Can you work these out from the model? Positions are in its coordinate system, mm. Face numbers are marked on the shaded views. A direction names the side the tool comes from. Coordinates: 2 decimals unless noted, no trailing zeros. Order: outer loops, then holes, each group sorted by start corner. A loop starts at its lowest first (then second) coordinate and runs counter-clockwise, first axis right, second up. Notation, with made-up numbers: (51, 4) -> (86, 4) arc R13 ccw to (86, 16) -> close; hole circle Ø8 at (33, 77.5). An arc over 180 degrees is marked (long way). Answer in a Markdown table with one row per item.
```python
from build123d import *

# Parameters (mm, degrees)
SKETCH1_W           = 80.5
SKETCH1_H           = 36.5
BOSS_EXTRUDE1_DEPTH = 1.6
SKETCH2_R           = 1.5
CUT_EXTRUDE1_DEPTH  = 1.6
SKETCH3_W           = 71.3
SKETCH3_H           = 26.799999994
BOSS_EXTRUDE2_DEPTH = 7.1
SKETCH4_R           = 0.5
CUT_EXTRUDE2_DEPTH  = 7.1
SKETCH5_W           = 64.5
SKETCH5_H           = 13.8
CUT_EXTRUDE3_DEPTH  = 1.5


with BuildPart() as part:
    # Sketch1 → Boss-Extrude1 (new body)
    with BuildSketch(Plane(origin=(0, 0, 0), x_dir=(1, 0, 0), z_dir=(0, 1, 0))):
        Rectangle(SKETCH1_W, SKETCH1_H)
    extrude(amount=BOSS_EXTRUDE1_DEPTH)

    # Sketch2 → Cut-Extrude1 (cut)
    with BuildSketch(Plane(origin=(0, 1.6, 0), x_dir=(1, 0, 0), z_dir=(0, 1, 0))):
        with Locations(Location((-37.75, 15.75, 0), (0, 0, 270))):
            Circle(SKETCH2_R)
        with Locations(Location((-37.75, -15.75, 0), (0, 0, 270))):
            Circle(SKETCH2_R)
        with Locations(Location((37.75, 15.75, 0), (0, 0, 270))):
            Circle(SKETCH2_R)
        with Locations(Location((37.75, -15.75, 0), (0, 0, 270))):
            Circle(SKETCH2_R)
    extrude(amount=-CUT_EXTRUDE1_DEPTH, mode=Mode.SUBTRACT)

    # Sketch3 → Boss-Extrude2 (add)
    with BuildSketch(Plane(origin=(0, 1.6, 0), x_dir=(1, 0, 0), z_dir=(0, 1, 0))):
        Rectangle(SKETCH3_W, SKETCH3_H)
    extrude(amount=BOSS_EXTRUDE2_DEPTH)

    # Sketch4 → Cut-Extrude2 (cut)
    with BuildSketch(Plane(origin=(0, 1.6, 0), x_dir=(1, 0, 0), z_dir=(0, 1, 0))):
        with Locations(Location((-32.25, 15.75, 0), (0, 0, 270))):
            Circle(SKETCH4_R)
        with Locations(Location((-29.71, 15.75, 0), (0, 0, 270))):
            Circle(SKETCH4_R)
        with Locations(Location((-27.17, 15.75, 0), (0, 0, 270))):
            Circle(SKETCH4_R)
        with Locations(Location((-24.63, 15.75, 0), (0, 0, 270))):
            Circle(SKETCH4_R)
        with Locations(Location((-22.09, 15.75, 0), (0, 0, 270))):
            Circle(SKETCH4_R)
        with Locations(Location((-19.55, 15.75, 0), (0, 0, 270))):
            Circle(SKETCH4_R)
        with Locations(Location((-17.01, 15.75, 0), (0, 0, 270))):
            Circle(SKETCH4_R)
        with Locations(Location((-14.47, 15.75, 0), (0, 0, 270))):
            Circle(SKETCH4_R)
        with Locations(Location((-11.93, 15.75, 0), (0, 0, 270))):
            Circle(SKETCH4_R)
        with Locations(Location((-9.39, 15.75, 0), (0, 0, 270))):
            Circle(SKETCH4_R)
        with Locations(Location((-6.85, 15.75, 0), (0, 0, 270))):
            Circle(SKETCH4_R)
        with Locations(Location((-4.31, 15.75, 0), (0, 0, 270))):
            Circle(SKETCH4_R)
        with Locations(Location((-1.77, 15.75, 0), (0, 0, 270))):
            Circle(SKETCH4_R)
        with Locations(Location((0.77, 15.75, 0), (0, 0, 270))):
            Circle(SKETCH4_R)
        with Locations(Location((3.31, 15.75, 0), (0, 0, 270))):
            Circle(SKETCH4_R)
        with Locations(Location((5.85, 15.75, 0), (0, 0, 270))):
            Circle(SKETCH4_R)
    extrude(amount=-CUT_EXTRUDE2_DEPTH, mode=Mode.SUBTRACT)

    # Sketch5 → Cut-Extrude3 (cut)
    with BuildSketch(Plane(origin=(0, 8.7, 0), x_dir=(1, 0, 0), z_dir=(0, 1, 0))):
        Rectangle(SKETCH5_W, SKETCH5_H)
    extrude(amount=-CUT_EXTRUDE3_DEPTH, mode=Mode.SUBTRACT)


solid = part.part
```
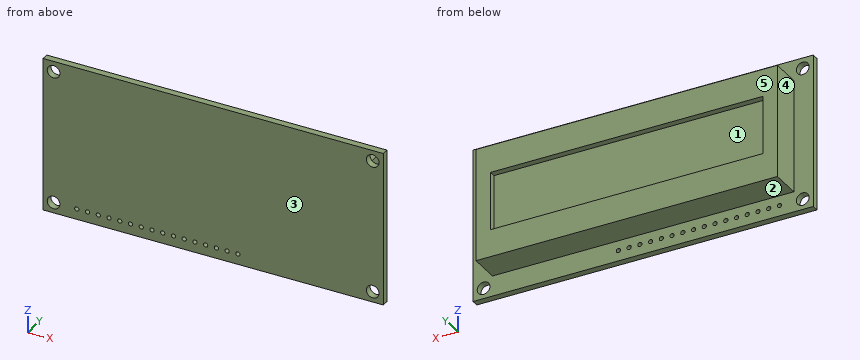
(1) Suppose I cut it at B-B (z = -10). Please give me the cut outline in (x, y), and give its area (3 significant figures).
Response values:
| item | result |
|---|---|
| outline | (-40.25, 0) -> (40.25, 0) -> (40.25, 1.6) -> (35.65, 1.6) -> (35.65, 8.7) -> (-35.65, 8.7) -> (-35.65, 1.6) -> (-40.25, 1.6) -> close |
| area | 635 mm2 |
(2) Suppose I cut it at A-A (x = -37.75). Please give me the cut outline in (y, z), and give its area (3 significant figures).
Response values:
| item | result |
|---|---|
| outline | (0, -18.25) -> (1.6, -18.25) -> (1.6, -17.25) -> (0, -17.25) -> close; (0, -14.25) -> (1.6, -14.25) -> (1.6, 14.25) -> (0, 14.25) -> close; (0, 17.25) -> (1.6, 17.25) -> (1.6, 18.25) -> (0, 18.25) -> close |
| area | 48.8 mm2 |
(3) Will these pins go through, and if not, where does the flat tip stop? pin 1 Ø5 at (y, z) = (6, 2) entering from -X; pin 2 Ø3.5 at (y, z) = (4, 4) entering from +X; pin 3 Ø2.5 at (x, z) = (-37.75, 15.75) entering from -Y; pin 4 Ø5 at (x, y) = (8, 7) entering from +Z.
Response values:
| item | result |
|---|---|
| pin 1 | x = -35.65 |
| pin 2 | x = 35.65 |
| pin 3 | through |
| pin 4 | z = 13.4 |
(4) Suppose I cut it at D-D (z = -6). Please give me the cut outline in (x, y), and give its area (3 significant figures).
Response values:
| item | result |
|---|---|
| outline | (-40.25, 0) -> (40.25, 0) -> (40.25, 1.6) -> (35.65, 1.6) -> (35.65, 8.7) -> (32.25, 8.7) -> (32.25, 7.2) -> (-32.25, 7.2) -> (-32.25, 8.7) -> (-35.65, 8.7) -> (-35.65, 1.6) -> (-40.25, 1.6) -> close |
| area | 538 mm2 |
(5) I need wall thicknesses on line 1 (X direction, y = 0.6, z = 15.75); line 2 (X direction, y = 7.75, z = -5); line 3 (Z direction, x = -0.5, y = 7.25). Which ranges of each line are inside material? Lowest first, please. Write a range as [from, to].
Response values:
| item | result |
|---|---|
| line 1 | [-40.25, -39.25], [-36.25, 36.25], [39.25, 40.25] |
| line 2 | [-35.65, -32.25], [32.25, 35.65] |
| line 3 | [-13.4, -6.9], [6.9, 13.4] |
(6) Suppose I cut it at C-C (y = 3). Please give me the cut outline in (x, z).
Response values:
| item | result |
|---|---|
| outline | (-35.65, -13.4) -> (35.65, -13.4) -> (35.65, 13.4) -> (-35.65, 13.4) -> close |
(7) On a 3-axis mill with a long thin cutter (end or side, diameter ignored), from which of +Z, -Z, +X, -X, +Y, -Y can I reach the whole of each face in a straight line? I mean the marked faces 4 and 5. Say none if no direction works.
Response values:
| item | result |
|---|---|
| face 4 | +Z, -Z, -X, +Y |
| face 5 | +Z, -Z, +X, -X, +Y |
(8) We'd pull the mould along Z, two halves only. Please class the marked faces 1, 2 and 3: +Z half, -Z half, draft (parallel to the pull), parting line (faces both ways), or undercut.
Response values:
| item | result |
|---|---|
| face 1 | undercut |
| face 2 | -Z half |
| face 3 | draft |
